from build123d import *

# Parameters (mm, degrees)
SKETCH_1_R      = 3
EXTRUDE_1_DEPTH = 3
FILLET_1_R      = 5


with BuildPart() as part:
    # ｽｹｯﾁ1 → ﾎﾞｽ - 押し出し1 (new body)
    with BuildSketch(Plane.XY):
        Polygon((-48.082594675, 5), (15.312222711, -64.010484178), (4.263144073, 5), align=None)
        with Locations((-36.7, 0)):
            Circle(SKETCH_1_R, mode=Mode.SUBTRACT)
        Circle(SKETCH_1_R, mode=Mode.SUBTRACT)
        with Locations((7.746594005, -48.38378118)):
            Circle(SKETCH_1_R, mode=Mode.SUBTRACT)
    extrude(amount=EXTRUDE_1_DEPTH)

    # ﾌｨﾚｯﾄ1
    fillet_1_edges = [part.edges().sort_by_distance(p)[0] for p in [
        (4.263144073, 5, 1.5),
        (15.312222711, -64.010484178, 1.5),
        (-48.082594675, 5, 1.5),
    ]]
    fillet(fillet_1_edges, radius=FILLET_1_R)


solid = part.part
The model under review builds one solid part; all positions refer to its coordinate system, in mm. Give positions to 0.01 mm unless a question says otherwise; leave off trailing zeros. Loops run counter-clockwise (first coordinate to the right, second up) from the corner with the lowest first, then second, coordinate; pieces in that order, holes last. Notation, with made-up numbers: (-19.75, -23) -> (-15.75, -23) arc R27 ccw to (-15.75, -7) -> close; hole circle Ø5 at (-20.75, -35.75). An arc over 180 degrees is marked (long way). Put each result on its own line as item: value. Start each with the question number.
1. Wall thickness on probe 1 along Y at (x, z) = (-34, 2.95); probe 2 along Y at (x, z) = (0, 2); probe 3 along Y at (x, z) = (-17, 1): over which ranges is each line inside the solid? List them lowest first.
2. Clearance check with flat-ended pins moving along their axes: P1, Ø9.5, axis at x = -36.7, y = 0, coming from the -Z side; P2, Ø1.5, axis at x = -27, z = 1.5, coming from the -Y side; P3, Ø1, axis at y = -41, z = 2, coming from the -X side; P4, Ø5.5, axis at x = 0, y = 0, coming from the -Z side. State where each tip first meets the part, or that it passes through.
3. We need section D-D on y = -21. State the section outline as (x, z) points.
4. We need section A-A on z = 1.25. State the section outline as (x, y) points, then the cut area to 3 significant figures.
5. Mouldability with a two-part tool opening along Y and no side actions: class faces 1 (the face through (-18, 5, 1)), 2 (the face through (-18.47, -27.236, 1.479)), 3 (the face through (-33.84, 0.9, 1.48)) as released by +Y, released by -Y, zero draft, split by the parting line, or undercut.
6. We need section B-B on x = 6.5. State the section outline as (y, z) points, then the cut area to 3 significant figures.
7. We need section C-C on y = 0. State the section outline as (x, z) points, then the cut area to 3 significant figures.
Determined:
1. probe 1: -10.33 to -1.31, 1.31 to 5
1. probe 2: -47.34 to -3, 3 to 5
1. probe 3: -28.84 to 5
2. P1: z = 0
2. P2: y = -18.77
2. P3: x = -6.29
2. P4: through
3. outline: (-24.2, 0) -> (8.43, 0) -> (8.43, 3) -> (-24.2, 3) -> close
4. outline: (-40.38, -3.38) -> (4.06, -51.77) arc R5 ccw to (12.68, -47.59) -> (4.94, 0.79) arc R5 ccw to (0, 5) -> (-36.7, 5) arc R5 ccw to start; hole circle Ø6 at (-36.7, 0); hole circle Ø6 at (0, 0); hole circle Ø6 at (7.75, -48.38)
4. area: 1,640 mm^2
5. face 1: released by +Y
5. face 2: released by -Y
5. face 3: undercut
6. outline: (-53.23, 0) -> (-51.11, 0) -> (-51.11, 3) -> (-53.23, 3) -> close; (-45.66, 0) -> (-8.97, 0) -> (-8.97, 3) -> (-45.66, 3) -> close
6. area: 116 mm^2
7. outline: (-41.7, 0) -> (-39.7, 0) -> (-39.7, 3) -> (-41.7, 3) -> close; (-33.7, 0) -> (-3, 0) -> (-3, 3) -> (-33.7, 3) -> close; (3, 0) -> (5.06, 0) -> (5.06, 3) -> (3, 3) -> close
7. area: 104 mm^2
